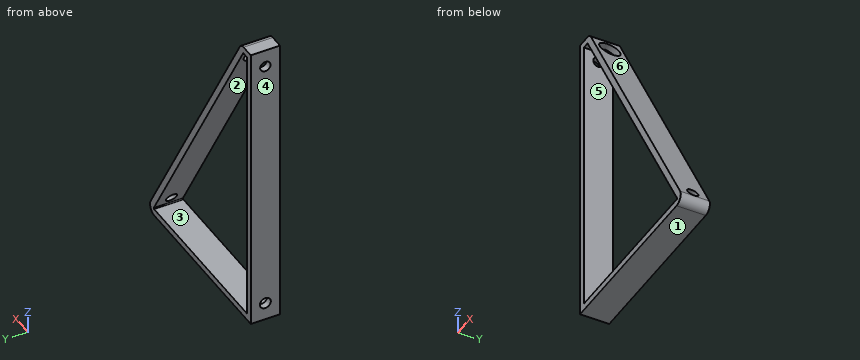
Autodesk Inventor part; units mm, degrees
ref_plane "YZ Plane" through (0, 0, 0) normal (1, 0, 0) x (0, 1, 0)
ref_plane "XZ Plane" through (0, 0, 0) normal (0, 1, 0) x (-1, 0, 0)
ref_plane "XY Plane" through (0, 0, 0) normal (0, 0, 1) x (1, 0, 0)
sketch "Náčrt1" plane through (0, 0, 0) normal (0, 1, 0) x (-1, 0, 0)
  line L0 (0, 0) -> (0, 83)
  line L1 (0, 83) -> (-2, 83)
  line L2 (-2, 83) -> (-49.9201, 0)
  line L3 (-49.9201, 0) -> (0, 0)
  line L4 (2, 85) -> (2, -2)
  line L5 (2, -2) -> (-53.3842, -2)
  line L6 (-53.3842, -2) -> (-3.1547, 85)
  line L7 (-3.1547, 85) -> (2, 85)
  dimension "d0" = 30
  dimension "d1" = 2
  dimension "d2" = 83
  dimension "d3" = 49.9201
  dimension "d4" = 2
extrude "Vysunutí1" add sketch "Náčrt1" along normal blind 8.5
sketch "Náčrt2" plane through (-2, 0, -2) normal (-1, 0, 0) x (0, 0, 1)
  line L0 (0, 0) -> (87, 0)
  line L1 (87, 0) -> (87, 8.5)
  line L2 (0, 8.5) -> (87, 8.5)
  line L3 (0, 0) -> (0, 8.5)
  line L4 (0, 4.25) -> (87, 4.25) construction
  circle A0 centre (5.2, 4.25) radius 1.5
  circle A1 centre (81.8, 4.25) radius 1.5
  line L5 (43.5, 8.5) -> (43.5, 0) construction
  circle A2 centre (5.2, 4.25) radius 3
  circle A3 centre (81.8, 4.25) radius 3
  point P0 (2, 0)
  dimension "d10" = 3
  dimension "d11" = 38.3
  dimension "d12" = 76.6
  dimension "d13" = 6
hole "Díra1" at (-2, 4.25, 79.8) at (-2, 4.25, 3.2) direction (1, 0, 0) diameter 3.2 end through all
extrude "Vysunutí2" cut sketch "Náčrt2" against normal blind 11.25 contours A3
extrude "Vysunutí3" add sketch "Náčrt2" against normal up to surface (2 mm away) contours A3
fillet "Zaoblení1" radius 2.25 2 edges at (53.3842, 4.25, -2) (3.1547, 4.25, 85)
fillet "Zaoblení1" radius 0.25 2 edges at (49.9201, 4.25, 0) (2, 4.25, 83)
properties part number "FL-LapTimer-Foot"
Part model, mm, in its own coordinate system. Face numbers are marked on the shaded views. A direction names the side the tool comes from. Give positions to 0.01 mm unless a question says otherwise; leave off trailing zeros. Loops run counter-clockwise (first coordinate to the right, second up) from the corner with the lowest first, then second, coordinate; pieces in that order, holes last. Notation, with made-up numbers: M -10,61.25 L 15,61.25 A25 cw 15,94.25 Z; hole C 53.25,45.25 d5. An arc over 180 degrees is marked long. Put each result on its own line as item: value. Start each with the question number.
1) Probe probe 1 along Z at (x, y) = (3.8, 4.25); probe 2 along Y at (x, z) = (49.5, 3); probe 3 along Y at (x, z) = (5.5, 79.8). List the from-to ranges inside material, lowest first.
2) 3-axis set-ups, long thin cutter, end or side, ignore diameter. For the marked faces 1 and 2: which of +Z, -Z, +X, -X, +Y, -Y reach the whole face in a straight line?
3) Flat gauge pins, fed straight in: pin 1 (3 mm diameter, centred on y = 4.25, z = 3.2, fed in from +X); pin 2 (3.5 mm diameter, centred on y = 4.25, z = 3.2, fed in from +X); pin 3 (4 mm diameter, centred on x = 19, y = 2, fed in from +Z); pin 4 (4 mm diameter, centred on y = 3.5, z = 45, fed in from +X). Where does each tip first touch, or does it go through?
4) Saw through at B-B (y = 4.25). List the corners of the cut face in (x, z) (3 decimals), then the cut area to 3 significant figures.
5) Saw through at D-D (z = 3.2). List the corners of the cut face in (x, y), then the cut area to 3 significant figures.
6) Pull direction Z, two halves, no side cores. Call the marked faces 3, 4, 5 and 6: +Z half, -Z half, draft (parallel to the pull), parting line (faces both ways), or undercut.
7) Saw through at C-C (x = 48.5). List the corners of the cut face in (y, z), then the cut area to 3 significant figures.
8) Saw through at A-A (z = 65). List the corners of the cut face in (x, y), then the cut area to 3 significant figures.
Numbers:
1. probe 1: -2 to 0, 82.8 to 83.88
1. probe 2: 0 to 2.66, 5.84 to 8.5
1. probe 3: 0 to 1.25, 7.25 to 8.5
2. face 1: -Z, +X, -X, +Y, -Y
2. face 2: +Y, -Y
3. pin 1: through
3. pin 2: x = 51.39
3. pin 3: z = 61.02
3. pin 4: x = 27.4
4. outline: M -2,-2 L 49.487,-2 A2.25 ccw 51.436,1.375 L 51.306,1.6 L 48.996,1.6 L 49.704,0.375 A0.25 cw 49.487,0 L 0,0 L 0,1.6 L -2,1.6 Z; M -2,4.8 L 0,4.8 L 0,78.3 L -2,78.3 Z; M -2,81.3 L 0,81.3 L 0,83 L 1.856,83 A0.25 cw 2.072,82.875 L 2.115,82.8 L 4.425,82.8 L 3.804,83.875 A2.25 ccw 1.856,85 L -2,85 Z; M 5.58,76.8 L 47.149,4.8 L 49.458,4.8 L 7.889,76.8 Z
4. area: 441 mm^2
5. outline: M -2,0 L 0,0 L 0,2.65 L -2,2.65 Z; M -2,5.85 L 0,5.85 L 0,8.5 L -2,8.5 Z; M 48.07,0 L 50.38,0 L 50.38,2.65 L 48.07,2.65 Z; M 48.07,5.85 L 50.38,5.85 L 50.38,8.5 L 48.07,8.5 Z
5. area: 22.8 mm^2
6. face 3: undercut
6. face 4: draft
6. face 5: undercut
6. face 6: +Z half
7. outline: M 0,-2 L 8.5,-2 L 8.5,0 L 0,0 Z; M 0,2.46 L 2.83,2.46 A1.6 cw long 5.67,2.46 L 8.5,2.46 L 8.5,6.46 L 0,6.46 Z
7. area: 44.7 mm^2
8. outline: M -2,0 L 0,0 L 0,8.5 L -2,8.5 Z; M 12.39,0 L 14.7,0 L 14.7,8.5 L 12.39,8.5 Z
8. area: 36.6 mm^2
